For this review, use the dimensioned drawing (mm, ordinates from the lowest corner) and the shaded views. A direction names the side the tool comes from. Round coordinates to 2 decimals unless told otherwise and drop trailing zeros. Loops run counter-clockwise (first coordinate to the right, second up) from the corner with the lowest first, then second, coordinate; pieces in that order, holes last. Notation, with made-up numbers: M 12.25,-2 L 41.25,-2 A23 ccw 41.25,11 Z; hole C 42.5,-18 d10. An arc over 180 degrees is marked long. Answer as a JSON object with one key per item and string values. Group by question number.
Item 1: Consider section A-A (x = 53). Give the boundary of the cut face in (y, z), and give its area (3 significant figures).
Item 2: Tool access review of the marked faces 1, 2, 3, 4 and 5: name each direction out of +Z, -Z, +X, -X, +Y, -Y from which nothing blocks a thin tool from reaching the whole face with its end or side.
Item 3: Insertion check: P1, Ø4, axis at y = 45.5, z = 18.5, coming from the -X side; P2, Ø7.5, axis at x = 53, z = 41, coming from the -Y side; P3, Ø6, axis at y = 26, z = 39, coming from the -X side; P4, Ø7.5, axis at y = 53.5, z = 38, coming from the +X side. Each pin has a flat end and moves straight along its axis. Give the tip position at first contact, or say it passes through.
Item 4: To check wall thickness, follow line 1 (Y direction, x = 42, z = 39.5); line 2 (Z direction, x = 46.5, y = 93.5). State the ranges of each line that lie inside material, in increasing order.
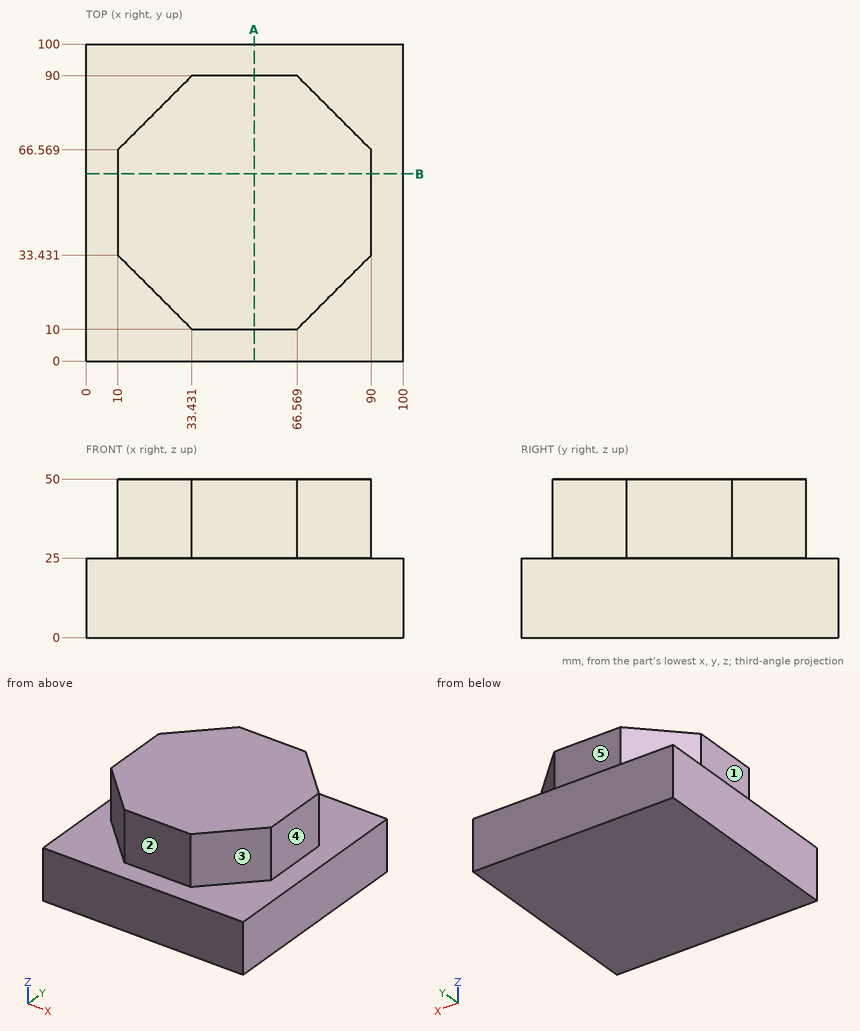
Geometry results:
{
 "1": {"outline": "M 0,0 L 100,0 L 100,25 L 90,25 L 90,50 L 10,50 L 10,25 L 0,25 Z", "area": "4,500 mm^2"},
 "2": {"face 1": "+Z, -X, +Y, -Y", "face 2": "+Z, +X, -X, -Y", "face 3": "+Z, +X, -Y", "face 4": "+Z, +X, +Y, -Y", "face 5": "+Z, +X, -X, +Y"},
 "3": {"P1": "stops at x = 0", "P2": "stops at y = 10", "P3": "stops at x = 14.43", "P4": "stops at x = 90"},
 "4": {"line 1": "y = 10 to 90", "line 2": "z = 0 to 25"}
}
